Autodesk Inventor part; units mm, degrees
ref_plane "YZ Plane" through (0, 0, 0) normal (1, 0, 0) x (0, 1, 0)
ref_plane "XZ Plane" through (0, 0, 0) normal (0, 1, 0) x (-1, 0, 0)
ref_plane "XY Plane" through (0, 0, 0) normal (0, 0, 1) x (1, 0, 0)
sketch "Sketch1" plane through (0, 0, 0) normal (0, 0, 1) x (1, 0, 0)
  line L0 (0, 0) -> (-5, 0)
  line L1 (-5, 0) -> (-5, 20)
  line L2 (-5, 20) -> (0, 20)
  line L3 (0, 20) -> (0, 0)
  arc A0 (0, 0) -> (3.7628, -11.2711) centre (16.9897, -0.5917) ccw
  arc A1 (-2.5, 0) -> (3.7698, -12.1977) centre (12.5, 0) ccw
  line L4 (4.0643, -12.4032) -> (3.7628, -11.2711)
  line L5 (-5, 0) -> (-2.5, 0)
  line L6 (0, 20) -> (0, 0)
  line L7 (3.7698, -12.1977) -> (4.0643, -12.4032)
  circle A2 centre (-3.75, 1.4711) radius 1.0155
  dimension "d0" = 5
  dimension "d1" = 20
  dimension "d2" = 17
  dimension "d3" = 15
extrude "Extrusion1" add sketch "Sketch1" against normal blind 13 contours L0 L1 L2 L3 | A2
extrude "Extrusion2" add sketch "Sketch1" against normal blind 1 contours A0 L4 L7 A1 L0
sketch "Sketch2" plane through (0, 0, -13) normal (1, 0, 0) x (0, 0, -1)
  line L0 (-12, 0) -> (0, 0)
  line L1 (-11, 14.4434) -> (-11, 18)
  line L2 (-2, 18) -> (-2, 0)
  line L3 (-2, 0) -> (-11, 0)
  line L4 (-13, 20) -> (0, 20)
  line L5 (-13, -11.2711) -> (-12, -11.2711)
  line L6 (-4.8653, 18) -> (-2, 18)
  line L7 (-13, 0) -> (-13, 20)
  line L8 (0, 20) -> (0, 0)
  line L9 (-11, 18) -> (-4.8653, 18)
  line L10 (-11, 14.4434) -> (-11, 0)
  line L11 (-13, 0) -> (0, 0)
  line L12 (-11, 20) -> (-11, 21.5)
  line L13 (-2, 21.5) -> (-2, 20)
  line L14 (-11, 20) -> (-2, 20)
  line L15 (-13, 20) -> (0, 20)
  line L16 (-6.5, 21.5) -> (-6.5, 20) construction
  line L17 (-5, 21.5) -> (-6.5, 20)
  line L18 (-6.5, 20) -> (-8, 21.5)
  line L19 (-2, 21.5) -> (-5, 21.5)
  line L20 (-8, 21.5) -> (-11, 21.5)
  point P0 (-1, 20)
  point P1 (-12, 20)
  point P2 (-12, 20.7344)
  point P3 (-2, 0)
  dimension "d10" = 18
  dimension "d19" = 2
  dimension "d20" = 2
  dimension "d24" = 2
  dimension "d25" = 4.5
  dimension "d26" = 2
  dimension "d27" = 1.5
  dimension "d28" = 1.5
extrude "Extrusion3" add sketch "Sketch2" against normal blind 5 contours L17 L19 L13 L4
extrude "Extrusion4" add sketch "Sketch2" against normal blind 5 contours L12 L20 L18 L4 | L17 L19 L13 L4
extrude "Extrusion5" cut sketch "Sketch2" against normal through all contours L10 L1 L9 L6 L2 L0
extrude "Extrusion6" cut sketch "Sketch1" against normal through all contours A2
fillet "Arredondamento1" radius 0.5 2 edges at (-2.5, 21.5, -11) (-2.5, 21.5, -2)
fillet "Arredondamento2" radius 0.5 2 edges at (-2.5, 20, -13) (-2.5, 20, 0)
sketch "Esboço3" plane through (-5, 0, -11) normal (-1, 0, 0) x (0, 0, 1)
  arc A0 (11, 19.5) -> (10.5, 20) centre (10.5, 19.5) ccw
  line L0 (10.5, 20) -> (9, 20)
  line L1 (9, 20) -> (9, 21)
  arc A1 (9, 21) -> (8.5, 21.5) centre (8.5, 21) ccw
  line L2 (8.5, 21.5) -> (6, 21.5)
  line L3 (6, 21.5) -> (4.5, 20)
  line L4 (4.5, 20) -> (3, 21.5)
  line L5 (3, 21.5) -> (0.5, 21.5)
  arc A2 (0.5, 21.5) -> (0, 21) centre (0.5, 21) ccw
  line L6 (0, 21) -> (0, 20)
  line L7 (0, 20) -> (-1.5, 20)
  arc A3 (-1.5, 20) -> (-2, 19.5) centre (-1.5, 19.5) ccw
  line L8 (-2, 0) -> (-2, 19.5)
  line L9 (0, 0) -> (-2, 0)
  line L10 (0, 0) -> (0, 18)
  line L11 (0, 18) -> (9, 18)
  line L12 (9, 18) -> (9, 0)
  line L13 (11, 0) -> (9, 0)
  line L14 (11, 19.5) -> (11, 0)
  point P0 (11, 0)
extrude "Extrusão7" add sketch "Esboço3" along normal blind 1
properties material "Nickel-Copper Alloy 400"
Could you check a few things on this model? Use its own coordinates, in mm. A direction names the side the tool comes from. Round coordinates to 2 decimals unless told otherwise and drop trailing zeros. Loops run counter-clockwise (first coordinate to the right, second up) from the corner with the lowest first, then second, coordinate; pieces in that order, holes last. Notation, with made-up numbers: M 65,-11.75 L 105,-11.75 A11 ccw 105,5.25 Z; hole C -40,-7 d4. An arc over 180 degrees is marked long. Answer as CSV lines item,"result".
1) Imagine slicing it at B-B on x = -3.75. List the corners of the cut face in (y, z) for me.
From the geometry:
outline,"M 0,-13 L 0.46,-13 L 0.46,-11 L 0,-11 Z; M 0,-2 L 0.46,-2 L 0.46,0 L 0,0 Z; M 2.49,-13 L 19.5,-13 A0.5 ccw 20,-12.5 L 20,-11 L 21,-11 A0.5 ccw 21.5,-10.5 L 21.5,-8 L 20,-6.5 L 21.5,-5 L 21.5,-2.5 A0.5 ccw 21,-2 L 20,-2 L 20,-0.5 A0.5 ccw 19.5,0 L 2.49,0 L 2.49,-2 L 18,-2 L 18,-11 L 2.49,-11 Z"
2) We'd pull the mould along X, two halves only. Please class faces 1 (the cylindrical face through (-4.498, 2.157, -11.986)), 2 (the flat face through (-3, 20.7, -7.2)), 3 (the flat face through (-6, 12.4, -11.3)), 4 (the flat face through (0, 12.4, -11.3)): released by +X, released by -X, zero draft, split by the parting line, or undercut.
From the geometry:
face 1,"undercut"
face 2,"zero draft"
face 3,"released by -X"
face 4,"released by +X"
3) If I drill on probe 1 along Y at (x, z) = (-3.75, -11.35); probe 2 along Z at (x, y) = (-2.5, 17.5); probe 3 along Z at (x, y) = (-1.25, -5), over which ranges is the centre line in solid material (lowest first)?
From the geometry:
probe 1,"0 to 0.46, 2.49 to 20"
probe 2,"-13 to -11, -2 to 0"
probe 3,"-1 to 0"
4) Imagine slicing it at A-A on y = 7.5. List the corners of the cut face in (x, z) for me, and give its area (3 significant figures).
From the geometry:
outline,"M -6,-13 L 0,-13 L 0,-11 L -6,-11 Z; M -6,-2 L 0,-2 L 0,0 L -6,0 Z"
area,"24.0 mm^2"
5) Imagine slicing it at C-C on x = -1. List the corners of the cut face in (y, z) for me.
From the geometry:
outline,"M -6.54,-1 L 0,-1 L 0,-2 L 18,-2 L 18,-11 L 0,-11 L 0,-13 L 19.5,-13 A0.5 ccw 20,-12.5 L 20,-11 L 21,-11 A0.5 ccw 21.5,-10.5 L 21.5,-8 L 20,-6.5 L 21.5,-5 L 21.5,-2.5 A0.5 ccw 21,-2 L 20,-2 L 20,-0.5 A0.5 ccw 19.5,0 L -6.54,0 Z"
6) Imagine slicing it at D-D on z = -3.5. List the corners of the cut face in (x, y) for me, and give its area (3 significant figures).
From the geometry:
outline,"M -6,18 L 0,18 L 0,21.5 L -6,21.5 Z"
area,"21.0 mm^2"
7) Which directions (+Z, -Z, +X, -X, +Y, -Y) give clear straight access to the entire face, cutting with the end or side of a thin tool? Please do faces 5 (the flat face through (-3, 18, -7)), 6 (the flat face through (-3, 0, -12)), 7 (the flat face through (-3, 20.8, -5.7)), 8 (the flat face through (-3, 20.5, -2)), 9 (the flat face through (-4, 0, -1)).
From the geometry:
face 5,"+X, -X, -Y"
face 6,"-Z, +X, -X, -Y"
face 7,"+X, -X, +Y"
face 8,"+Z, +X, -X, +Y"
face 9,"-Z, -X, -Y"
8) For pin 1 Ø5.5 at (x, y) = (-0.5, -4.5) entering from -Z; pin 2 Ø0.8 at (x, z) = (-2, -11.5) entering from +Y; pin 3 Ø5 at (x, z) = (-3, -5) entering from -Y; pin 4 Ø1.8 at (x, y) = (-3.5, 11) entering from +Z, each with a flat end and sliding along its axis, tell me the tip position at first contact or that it passes through.
From the geometry:
pin 1,"z = -1"
pin 2,"y = 20"
pin 3,"y = 18"
pin 4,"z = 0"
